The listing builds one solid part. Answer for the finished solid, in the listing's coordinates (mm). A direction names the side the tool comes from. Round coordinates to 2 decimals unless told otherwise and drop trailing zeros. Write each loop counter-clockwise with the first axis right and the second up, starting at its lowest first coordinate (ties: lowest second). Pieces come first, ordered by that corner, then holes.
Item 1: Find section C-C on x = -37.5. Give the vertices of the cut face in (y, z), then the cut area to 3 significant figures.
Item 2: A tool of negligible diameter and unlimited length cuts with its end or side. For faces 1 (the face through (-2.843, -12.804, 46.659)), 2 (the face through (-1, 38.1, 10)), 3 (the face through (-5.506, -24.796, 34.564)), from which of +Z, -Z, +X, -X, +Y, -Y can it reach the whole face along a straight path? Write none if from no direction.
Item 3: Find section A-A on x = -66.04. Give the vertices of the cut face in (y, z), then the cut area to 3 significant figures.
Item 4: Find section B-B on y = 0. Give the vertices of the cut face in (x, z), then the cut area to 3 significant figures.
Item 5: Find section D-D on z = 49. Give the vertices of the cut face in (x, y).
Item 6: For a pull along X with two mould halves and no side action, classify faces 4 (the face through (74.19, 0.53, 22.33)), 5 (the face through (60.676, 25.907, 12.878)), 6 (the face through (0, 0, 76.2)) as +X half, -X half, draft (parallel to the pull), parting line (faces both ways), or undercut.
Item 7: Each of these flat-tipped pins is pushed along its axis until it touches: pin 1 (4 mm diameter, centred on y = 10.5, z = 58, fed in from -X); pin 2 (4 mm diameter, centred on x = 52.5, z = 22.5, fed in from +Y); pin 3 (6 mm diameter, centred on y = -26.5, z = 64.5, fed in from +X). Where does it stop, or does it pass through?
Item 8: Find the intervals of material crossed by probe 1 along X at (y, z) = (25.5, 5); probe 2 along Y at (x, z) = (-66, 6); probe 3 along X at (y, z) = (-27, 14), in increasing order.
```python
from build123d import *

# Parameters (mm, degrees)
F0_W         = 152.4
F0_H         = 76.2
F1_DEPTH     = 25.4
F2_R         = 7.0539826123
F3_DEPTH     = 25.401
F4_W         = 25.4
F4_H         = 50.8
F6_W         = 18.2314971462
F6_H         = 16.024235636
F9_R         = 5.08
F10_T1_DEPTH = 178.5282991577
F10_T3_DEPTH = 102.3282991577


# Not quite as in the source:
# - a fillet or chamfer that OpenCascade refuses, or shapes differently, is made with other operations: its cross-section is extruded or revolved along the edge and cut away or added


with BuildPart() as f1:
    # F0 (on Top) → F1 (new body)
    with BuildSketch(Plane.XY):
        Rectangle(F0_W, F0_H)
    extrude(amount=F1_DEPTH)

    # F2 (on face) → F3 (cut, through all)
    with BuildSketch(Plane.XY.offset(25.4)):
        with Locations((67.723274231, 25.5973488092)):
            Circle(F2_R)
        with Locations((-66.04, 25.5973488092)):
            Circle(F2_R)
        with Locations((-66.04, -27.94)):
            Circle(F2_R)
        with Locations((67.723274231, -27.94)):
            Circle(F2_R)
    extrude(amount=-F3_DEPTH, mode=Mode.SUBTRACT)

    # F4 (on Front) → F5 (revolve)
    with BuildSketch(Plane.XZ):
        with Locations((12.7, 50.8)):
            Rectangle(F4_W, F4_H)
    revolve(axis=Axis((0, 0, 50.8), (0, 0, 1)))

    # F6 (on Front) → F8 (revolve, cut)
    with BuildSketch(Plane.XZ):
        with Locations((22.2315485589, 46.5468037874)):
            Rectangle(F6_W, F6_H)
    revolve(axis=Axis((0, 0, 32.2526581585), (0, 0, 1)), mode=Mode.SUBTRACT)

    # F9
    f9_edges = [f1.edges().sort_by_distance(p)[0] for p in [
        (-25.4, 0, 76.2),
        (-25.4, 0, 25.4),
    ]]
    fillet(f9_edges, radius=F9_R)

    # F10: chamfer of 5.08 on 4 edges, made by hand

    # F10_s2 → F10_t1 (cut)
    with BuildSketch(Plane.YZ.offset(-89.2641495789)):
        Polygon((-33.02, 25.4), (-38.1, 20.32), (-38.1, 25.4), align=None)
        Polygon((33.02, 25.4), (38.1, 20.32), (38.1, 25.4), align=None)
    extrude(amount=F10_T1_DEPTH, mode=Mode.SUBTRACT)

    # F10_s4 → F10_t3 (cut)
    with BuildSketch(Plane.XZ.offset(-51.1641495789)):
        Polygon((71.12, 25.4), (76.2, 20.32), (76.2, 25.4), align=None)
        Polygon((-71.12, 25.4), (-76.2, 20.32), (-76.2, 25.4), align=None)
    extrude(amount=F10_T3_DEPTH, mode=Mode.SUBTRACT)


solid = f1.part
```
Check values:
1. outline: (-38.1, 0) - (38.1, 0) - (38.1, 20.32) - (33.02, 25.4) - (-33.02, 25.4) - (-38.1, 20.32) - close
1. area: 1,910 mm2
2. face 1: none
2. face 2: +Z, -Z, +X, -X, +Y
2. face 3: +Z
3. outline: (-38.1, 0) - (-34.99, 0) - (-34.99, 23.43) - (-38.1, 20.32) - close; (-20.89, 0) - (18.54, 0) - (18.54, 25.4) - (-20.89, 25.4) - close; (32.65, 0) - (38.1, 0) - (38.1, 20.32) - (33.02, 25.4) - (32.65, 25.4) - close
3. area: 1,190 mm2
4. outline: (-76.2, 0) - (76.2, 0) - (76.2, 20.32) - (71.12, 25.4) - (30.48, 25.4) arc R5.08 cw to (25.4, 30.48) - (25.4, 38.53) - (13.12, 38.53) - (13.12, 54.56) - (25.4, 54.56) - (25.4, 71.12) arc R5.08 ccw to (20.32, 76.2) - (-20.32, 76.2) arc R5.08 ccw to (-25.4, 71.12) - (-25.4, 54.56) - (-13.12, 54.56) - (-13.12, 38.53) - (-25.4, 38.53) - (-25.4, 30.48) arc R5.08 cw to (-30.48, 25.4) - (-71.12, 25.4) - (-76.2, 20.32) - close
4. area: 6,030 mm2
5. outline: circle Ø26.23 at (0, 0)
6. face 4: +X half
6. face 5: undercut
6. face 6: draft
7. pin 1: stops at x = -23.94
7. pin 2: stops at y = 37.92
7. pin 3: stops at x = 9.64
8. probe 1: x = -76.2 to -73.09, -58.99 to 60.67, 74.78 to 76.2
8. probe 2: y = -38.1 to -34.99, -20.89 to 18.54, 32.65 to 38.1
8. probe 3: x = -76.2 to -73.03, -59.05 to 60.73, 74.71 to 76.2
